Could you check a few things on this drawing? It's one solid part, dimensions in mm from its lowest x, y, z. Coordinates: 2 decimals unless noted, no trailing zeros. Loops run counter-clockwise (first coordinate to the right, second up) from the corner with the lowest first, then second, coordinate; pieces in that order, holes last.
1) Imagine slicing it at B-B on x = 108.7. Please give me the cut outline in (y, z), plus the area to 3 significant figures.
2) Will these pins go through, and if not, where does the flat tip stop? P1, Ø4, axis at x = 113.5, z = 11, coming from the +Y side; P2, Ø19, axis at x = 43.7, y = 19.91, coming from the -Z side; P3, Ø2, axis at y = 17, z = 3, coming from the -X side (1 decimal); P4, Ø4, axis at x = 84.5, y = 75.5, coming from the +Z side.
3) Thinking about a two-plate mould opening in X: for the marked faces 1, 2 and 3, which applies, released by +X, released by -X, zero draft, split by the parting line, or undercut?
4) Imagine slicing it at C-C on y = 22. Please give me the cut outline in (x, z).
5) If I drill on line 1 along X through (y, z) = (134.5, 6) (1 decimal); line 2 along Y through (x, z) = (108.7, 8.25); line 3 along Y through (x, z) = (109.5, 6) (1 decimal), over which ranges is the centre line in solid material (lowest first)?
6) Imagine slicing it at D-D on x = 12.5. Please give me the cut outline in (y, z).
7) Imagine slicing it at A-A on z = 3.25. Please give me the cut outline in (x, y).
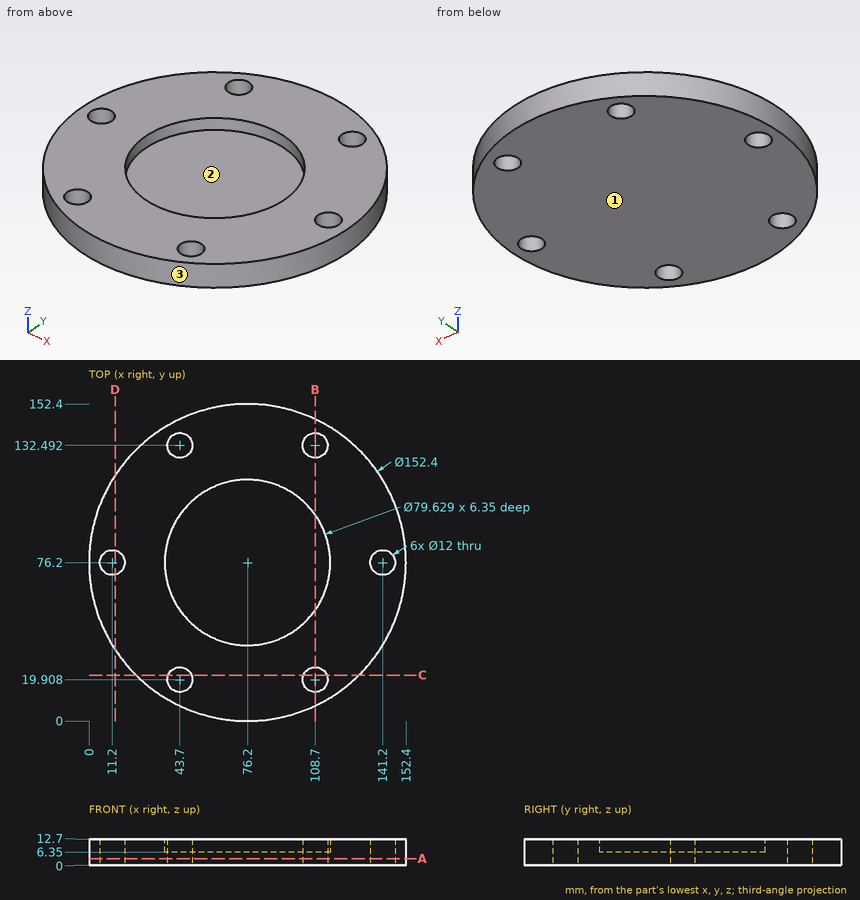
Filled in:
1. outline: (7.28, 0) - (13.91, 0) - (13.91, 12.7) - (7.28, 12.7) - close; (25.91, 0) - (126.49, 0) - (126.49, 12.7) - (99.2, 12.7) - (99.2, 6.35) - (53.2, 6.35) - (53.2, 12.7) - (25.91, 12.7) - close; (138.49, 0) - (145.12, 0) - (145.12, 12.7) - (138.49, 12.7) - close
1. area: 1,150 mm2
2. P1: stops at y = 143.73
2. P2: stops at z = 0
2. P3: stops at x = 27
2. P4: stops at z = 6.35
3. face 1: zero draft
3. face 2: undercut
3. face 3: split by the parting line
4. outline: (22.64, 0) - (38.08, 0) - (38.08, 12.7) - (22.64, 12.7) - close; (49.32, 0) - (103.08, 0) - (103.08, 12.7) - (49.32, 12.7) - close; (114.32, 0) - (129.76, 0) - (129.76, 12.7) - (114.32, 12.7) - close
5. line 1: x = 27.1 to 38, 49.4 to 103, 114.4 to 125.3
5. line 2: y = 7.28 to 13.91, 25.91 to 53.2, 99.2 to 126.49, 138.49 to 145.12
5. line 3: y = 7.7 to 14, 25.9 to 126.5, 138.4 to 144.7
6. outline: (34.38, 0) - (70.34, 0) - (70.34, 12.7) - (34.38, 12.7) - close; (82.06, 0) - (118.02, 0) - (118.02, 12.7) - (82.06, 12.7) - close
7. outline: circle Ø152.4 at (76.2, 76.2); hole circle Ø12 at (11.2, 76.2); hole circle Ø12 at (43.7, 19.91); hole circle Ø12 at (43.7, 132.49); hole circle Ø12 at (108.7, 19.91); hole circle Ø12 at (108.7, 132.49); hole circle Ø12 at (141.2, 76.2)
